CAD build for the part. Positions are in the model's coordinates, mm. Face numbers are marked on the shaded views. A direction names the side the tool comes from. Give positions to 0.01 mm unless a question says otherwise; leave off trailing zeros. Loops run counter-clockwise (first coordinate to the right, second up) from the corner with the lowest first, then second, coordinate; pieces in that order, holes last.
Item 1: Which spindle directions (+Z, -Z, +X, -X, +Y, -Y) get a long thin tool onto all of the face, cutting with end or side? Do the marked faces 1 and 2. Say none if no direction does.
Item 2: Saw through at B-B on y = 57. Give the cut face in (x, z).
Item 3: Saw through at A-A on x = 112.5. Give the cut face in (y, z).
Item 4: Drop flat-ended pins along their axis: P1, Ø5, axis at y = 51, z = 0, coming from the +X side; P2, Ø3, axis at y = 22.5, z = 5.5, coming from the +X side; P3, Ø2, axis at x = 18.5, z = 8, coming from the -Y side. Give the stop position or say it passes through.
Item 5: Probe probe 1 along X at (y, z) = (6, 5); probe 2 along X at (y, z) = (10, 1); probe 3 along Y at (x, z) = (137.5, 5.75). List the from-to ranges inside material, lowest first.
Item 6: Mould opens along X. For the marked faces 3 and 4 say: released by +X, released by -X, zero draft, split by the parting line, or undercut.
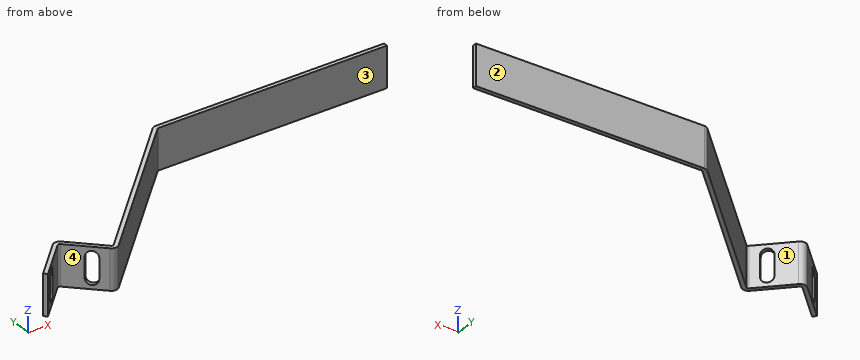
from build123d import *

# Parameters (mm, degrees)
BASE_FLANGE1_DEPTH = 10
CUT_EXTRUDE1_DEPTH = 2.032
CUT_EXTRUDE2_DEPTH = 2.032


# Sheet-metal steps are written as plain solids
with BuildPart() as part:
    # Sketch1 → Base-Flange1 (new, symmetric)
    with BuildSketch(Plane.XY):
        with BuildLine():
            Line((-17.225320151, -6), (-0.707106781, 10.51821337))
            ThreePointArc((-0.707106781, 10.51821337), (0, 10.811106589), (0.707106781, 10.51821337))
            Line((0.707106781, 10.51821337), (15.081372391, -3.856052239))
            ThreePointArc((15.081372391, -3.856052239), (17.225320151, -4.744104479), (19.369267912, -3.856052239))
            Line((19.369267912, -3.856052239), (85.932426933, 62.707106781))
            ThreePointArc((85.932426933, 62.707106781), (86.256850281, 62.923879533), (86.639533714, 63))
            Line((86.639533714, 63), (200, 63))
            Line((200, 63), (200, 65.032))
            Line((200, 65.032), (86.639533714, 65.032))
            ThreePointArc((86.639533714, 65.032), (85.479237547, 64.801202743), (84.495585953, 64.143947761))
            Line((84.495585953, 64.143947761), (17.932426933, -2.41921126))
            ThreePointArc((17.932426933, -2.41921126), (17.225320151, -2.712104479), (16.51821337, -2.41921126))
            Line((16.51821337, -2.41921126), (2.143947761, 11.95505435))
            ThreePointArc((2.143947761, 11.95505435), (0, 12.843106589), (-2.143947761, 11.95505435))
            Line((-2.143947761, 11.95505435), (-18.662161131, -4.563159021))
            Line((-18.662161131, -4.563159021), (-17.225320151, -6))
        make_face()
    extrude(amount=BASE_FLANGE1_DEPTH, both=True)

    # Sketch6 → Cut-Extrude1 (cut)
    with BuildSketch(Plane(origin=(-7.049501055, 7.049501055, 0), x_dir=(0, 0, 1), z_dir=(-0.7071067811865488, 0.7071067811865464, 0))):
        with BuildLine():
            Line((-5, -5), (5, -5))
            ThreePointArc((5, -5), (8, -8), (5, -11))
            Line((5, -11), (-5, -11))
            ThreePointArc((-5, -11), (-8, -8), (-5, -5))
        make_face()
    extrude(amount=-CUT_EXTRUDE1_DEPTH, mode=Mode.SUBTRACT)

    # Sketch9 → Cut-Extrude2 (cut)
    with BuildSketch(Plane(origin=(7.049501055, 7.049501055, 0), x_dir=(0, 0, -1), z_dir=(0.7071067811865488, 0.7071067811865464, 0))):
        with BuildLine():
            Line((-5, -3), (5, -3))
            ThreePointArc((5, -3), (8, -6), (5, -9))
            Line((5, -9), (-5, -9))
            ThreePointArc((-5, -9), (-8, -6), (-5, -3))
        make_face()
    extrude(amount=-CUT_EXTRUDE2_DEPTH, mode=Mode.SUBTRACT)


solid = part.part
Results below:
1. face 1: +Z, -Z, +Y
1. face 2: +Z, -Z, +X, -X, +Y
2. outline: (77.35, -10) - (80.23, -10) - (80.23, 10) - (77.35, 10) - close
3. outline: (63, -10) - (65.03, -10) - (65.03, 10) - (63, 10) - close
4. P1: stops at x = 76.73
4. P2: stops at x = 47.23
4. P3: stops at y = -4.73
5. probe 1: x = -8.1 to -5.23, 5.23 to 8.1, 26.35 to 29.23
5. probe 2: x = -4.1 to -1.23, 1.23 to 4.1, 30.35 to 33.23
5. probe 3: y = 63 to 65.03
6. face 3: zero draft
6. face 4: undercut
